Can you work these out from the drawing? Everything is in mm from the part's minimum corner. Coordinates: 2 decimals unless noted, no trailing zeros. Order: outer loops, then holes, each group sorted by start corner. A loop starts at its lowest first (then second) coordinate and runs counter-clockwise, first axis right, second up. Notation, with made-up numbers: (-30.75, 35.5) - (-9.75, 35.5) arc R26 ccw to (-9.75, 60.5) - close; hole circle Ø5 at (56, 22). An arc over 180 degrees is marked (long way). Answer as CSV lines item,"result". Start each with the question number.
Item 1: I'm going to push flat-ended pins straight in: pin 1 (4.5 mm diameter, centred on x = 63, z = 113, fed in from -Y); pin 2 (3 mm diameter, centred on x = 59, z = 28, fed in from -Y). Where does each tip first touch, or does it pass through?
Item 2: Imagine slicing it at A-A on x = 17.5. List the corners of the cut face in (y, z) for me, and give its area (3 significant figures).
Item 3: I need wall thicknesses on line 1 (X direction, y = 0.6, z = 70); line 2 (Z direction, x = 32.5, y = 1.6); line 3 (Z direction, x = 62.5, y = 1.3). Which ranges of each line are inside material? Lowest first, please.
Item 4: Imagine slicing it at B-B on z = 96. List the corners of the cut face in (x, y) for me, and give its area (3 significant figures).
Item 5: Imagine slicing it at D-D on y = 2.05. Count the separate pieces of the cut face and the enclosed holes in it, and give its area (3 significant figures).
Item 6: Imagine slicing it at C-C on x = 26.5. List the corners of the cut face in (y, z) for me, and give its area (3 significant figures).
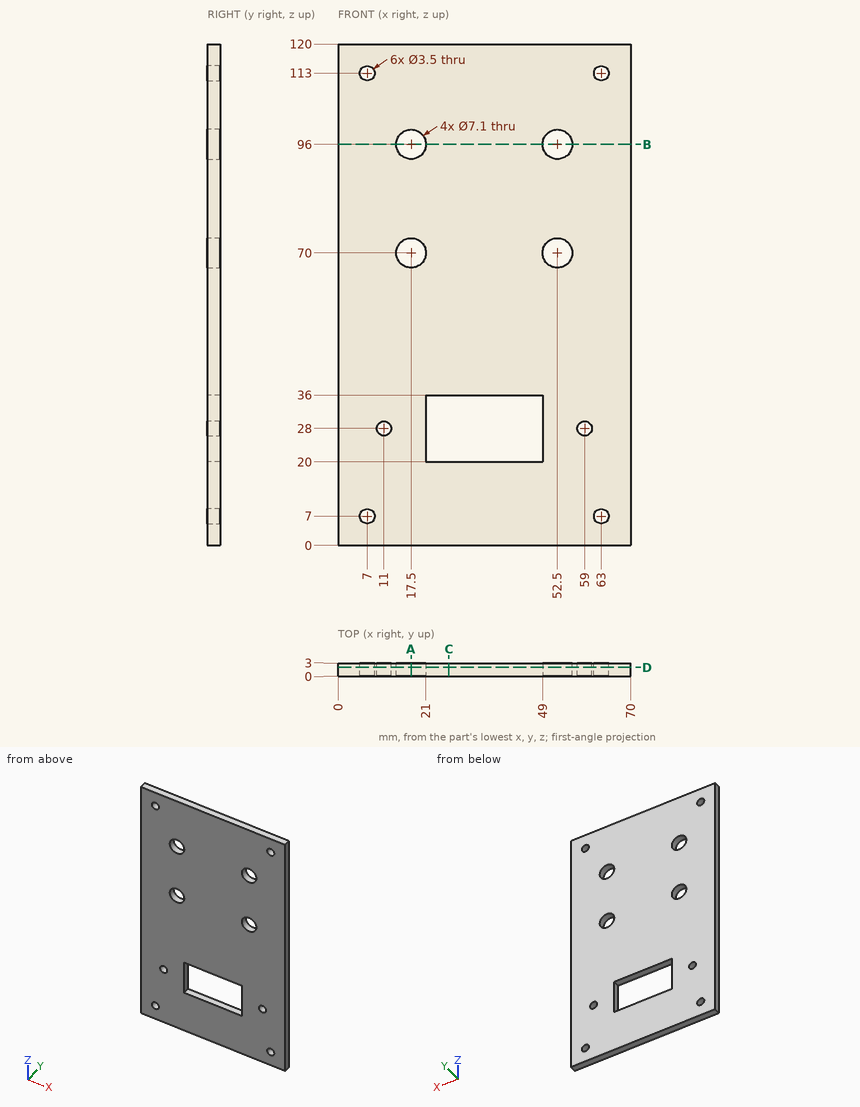
Responses:
1,pin 1,"stops at y = 0"
1,pin 2,"passes through"
2,outline,"(0, 0) - (3, 0) - (3, 66.45) - (0, 66.45) - close; (0, 73.55) - (3, 73.55) - (3, 92.45) - (0, 92.45) - close; (0, 99.55) - (3, 99.55) - (3, 120) - (0, 120) - close"
2,area,"317 mm^2"
3,line 1,"x = 0 to 13.95, 21.05 to 48.95, 56.05 to 70"
3,line 2,"z = 0 to 20, 36 to 120"
3,line 3,"z = 0 to 5.32, 8.68 to 111.32, 114.68 to 120"
4,outline,"(0, 0) - (13.95, 0) - (13.95, 3) - (0, 3) - close; (21.05, 0) - (48.95, 0) - (48.95, 3) - (21.05, 3) - close; (56.05, 0) - (70, 0) - (70, 3) - (56.05, 3) - close"
4,area,"167 mm^2"
5,separate pieces,"1"
5,enclosed holes,"11"
5,area,"7,740 mm^2"
6,outline,"(0, 0) - (3, 0) - (3, 20) - (0, 20) - close; (0, 36) - (3, 36) - (3, 120) - (0, 120) - close"
6,area,"312 mm^2"
